Input: part model. Units: mm. Frame: model coordinates. A direction names the side the tool comes from. Give positions to 0.01 mm unless a question says otherwise; leave off trailing zeros. Write each loop counter-clockwise with the first axis right and the second up, starting at its lowest first coordinate (ties: lowest second). Pieces come first, ordered by that corner, then holes. Notation, with made-up numbers: (60, -21.75) - (118, -21.75) arc R23 ccw to (118, 8.25) - close; hole circle Ø3 at (54, -16.5). An arc over 180 degrees is marked (long way). Use a Markdown table: item, result. Add a question column.
1. Mould query, pull axis X, two halves, no side actions, for faces 6 (the flat face through (123, 28, 39)), 7 (the flat face through (103.5, 15, 0)), 8 (the cylindrical face through (25, 15, -31)). Classes: released by +X, released by -X, zero draft, split by the parting line, or undercut.
2. Section query D-D, the plane x = 56.5. Return loops of the section in (y, z).
3. Material intervals for probe 1 along Z at (x, y) = (79.5, 19.25); probe 2 along Z at (x, y) = (112, 23.5); probe 3 along Y at (x, z) = (31, -23), sorted ascending.
4. Section query A-A, the plane x = 110. Return loops of the section in (y, z).
5. Section query B-B, the plane y = 22.75. Return loops of the section in (x, z), plus the area to 3 significant figures.
6. Pin query (flat end, axial travel): pin 1 (4 mm diameter, centred on y = 23, z = 14.5, fed in from +X); pin 2 (9 mm diameter, centred on y = 25, z = 15, fed in from -X); pin 3 (10.5 mm diameter, centred on x = 56.5, z = -32, fed in from +Y); pin 4 (8 mm diameter, centred on x = 70, z = -30, fed in from +Y). Return the tip coordinate at first contact, or that it passes through.
7. Set-up query: faces 1 (the flat face through (71, 15, -48)), 2 (the flat face through (56, 15, 36.5)), 3 (the flat face through (105, 4, -39)), 4 (the flat face through (119, 26, -31)), 5 (the flat face through (119, 4, -31)). Return all of +Z, -Z, +X, -X, +Y, -Y with unobstructed straight access to the full face (end or side cutting, diameter ignored); none if empty.
8. Section query C-C, the plane z = -5.5. Return loops of the section in (x, y), plus the area to 3 significant figures.
```python
from build123d import *

# Parameters (mm, degrees)
BOSS_EXTRUDE1_DEPTH = 30
CUT_EXTRUDE1_DEPTH  = 2
CUT_EXTRUDE2_DEPTH  = 2
SKETCH5_W           = 6.5
SKETCH5_H           = 96
CUT_EXTRUDE3_DEPTH  = 11.5
CUT_EXTRUDE4_DEPTH  = 5.5
CUT_EXTRUDE5_DEPTH  = 5.5
SKETCH8_W           = 25
SKETCH8_H           = 30
CUT_EXTRUDE6_DEPTH  = 1
SKETCH9_W           = 25
SKETCH9_H           = 30
CUT_EXTRUDE7_DEPTH  = 0.5


with BuildPart() as part:
    # Sketch2 → Boss-Extrude1 (new body)
    # profile 1 of 3: a face of its own
    with BuildSketch(Plane(origin=(0, 0, 0), x_dir=(1, 0, 0), z_dir=(0, 1, 0))):
        Polygon((114.5, 12.5), (133, 31), (98, 31), (98, 48), (0, 48), (0, -48), (98, -48), (98, -31), (133, -31), (114.5, -12.5), (105, -12.5), (105, 12.5), align=None)
        with BuildLine():
            Line((81.5, -36.5), (30.5, -36.5))
            ThreePointArc((30.5, -36.5), (25, -31), (30.5, -25.5))
            Line((30.5, -25.5), (81.5, -25.5))
            ThreePointArc((81.5, -25.5), (87, -31), (81.5, -36.5))
        make_face(mode=Mode.SUBTRACT)
        with BuildLine():
            ThreePointArc((30.5, 25.5), (25, 31), (30.5, 36.5))
            Line((30.5, 36.5), (81.5, 36.5))
            ThreePointArc((81.5, 36.5), (87, 31), (81.5, 25.5))
            Line((81.5, 25.5), (30.5, 25.5))
        make_face(mode=Mode.SUBTRACT)
    # profile 2 of 3: a face of its own
    with BuildSketch(Plane(origin=(0, 0, 0), x_dir=(1, 0, 0), z_dir=(0, 1, 0))):
        Polygon((133, 31), (140, 38), (140, 48), (98, 48), (98, 31), align=None)
    # profile 3 of 3: a face of its own
    with BuildSketch(Plane(origin=(0, 0, 0), x_dir=(1, 0, 0), z_dir=(0, 1, 0))):
        Polygon((98, -31), (98, -48), (140, -48), (140, -38), (133, -31), align=None)
    extrude(amount=BOSS_EXTRUDE1_DEPTH)

    # Sketch3 → Cut-Extrude1 (cut)
    with BuildSketch(Plane(origin=(0, 30, 0), x_dir=(1, 0, 0), z_dir=(0, 1, 0))):
        Polygon((105, 48), (105, 31), (133, 31), (140, 38), (140, 48), align=None)
        Polygon((140, -38), (140, -48), (105, -48), (105, -31), (133, -31), align=None)
    extrude(amount=-CUT_EXTRUDE1_DEPTH, mode=Mode.SUBTRACT)

    # Sketch4 → Cut-Extrude2 (cut)
    with BuildSketch(Plane.XZ):
        Polygon((105, 48), (105, 31), (133, 31), (140, 38), (140, 48), align=None)
        Polygon((105, -48), (105, -31), (133, -31), (140, -38), (140, -48), align=None)
    extrude(amount=-CUT_EXTRUDE2_DEPTH, mode=Mode.SUBTRACT)

    # Sketch5 → Cut-Extrude3 (cut)
    with BuildSketch(Plane(origin=(0, 30, 0), x_dir=(1, 0, 0), z_dir=(0, 1, 0))):
        with Locations((3.25, 0)):
            Rectangle(SKETCH5_W, SKETCH5_H)
    extrude(amount=-CUT_EXTRUDE3_DEPTH, mode=Mode.SUBTRACT)

    # Sketch6 → Cut-Extrude4 (cut)
    with BuildSketch(Plane(origin=(0, 30, 0), x_dir=(1, 0, 0), z_dir=(0, 1, 0))):
        Polygon((105, 12.5), (6.5, 12.5), (6.5, 48), (105, 48), (105, 31), (133, 31), (114.5, 12.5), align=None)
        Polygon((105, -12.5), (6.5, -12.5), (6.5, -48), (105, -48), (105, -31), (133, -31), (114.5, -12.5), align=None)
    extrude(amount=-CUT_EXTRUDE4_DEPTH, mode=Mode.SUBTRACT)

    # Sketch7 → Cut-Extrude5 (cut)
    with BuildSketch(Plane.XZ):
        Polygon((105, 12.5), (6.5, 12.5), (6.5, -12.5), (105, -12.5), (114.5, -12.5), (133, -31), (105, -31), (105, -48), (0, -48), (0, 48), (105, 48), (105, 31), (133, 31), (114.5, 12.5), align=None)
    extrude(amount=-CUT_EXTRUDE5_DEPTH, mode=Mode.SUBTRACT)

    # Sketch8 → Cut-Extrude6 (cut)
    with BuildSketch(Plane(origin=(105, 0, 0), x_dir=(0, 0, -1), z_dir=(1, 0, 0))):
        with Locations((0, 15)):
            Rectangle(SKETCH8_W, SKETCH8_H)
    extrude(amount=-CUT_EXTRUDE6_DEPTH, mode=Mode.SUBTRACT)

    # Sketch9 → Cut-Extrude7 (cut)
    with BuildSketch(Plane(origin=(104, 0, 0), x_dir=(0, 0, -1), z_dir=(1, 0, 0))):
        with Locations((0, 15)):
            Rectangle(SKETCH9_W, SKETCH9_H)
    extrude(amount=-CUT_EXTRUDE7_DEPTH, mode=Mode.SUBTRACT)


solid = part.part
```
Result sheet:
| question | item | result |
|---|---|---|
| 1 | face 6 | zero draft |
| 1 | face 7 | released by +X |
| 1 | face 8 | undercut |
| 2 | outline | (0, -12.5) - (5.5, -12.5) - (5.5, -25.5) - (24.5, -25.5) - (24.5, -12.5) - (30, -12.5) - (30, 12.5) - (24.5, 12.5) - (24.5, 25.5) - (5.5, 25.5) - (5.5, 12.5) - (0, 12.5) - close; (5.5, -48) - (24.5, -48) - (24.5, -36.5) - (5.5, -36.5) - close; (5.5, 36.5) - (24.5, 36.5) - (24.5, 48) - (5.5, 48) - close |
| 3 | probe 1 | z = -48 to -36.5, -25.5 to 25.5, 36.5 to 48 |
| 3 | probe 2 | z = -48 to -12.5, 12.5 to 48 |
| 3 | probe 3 | y = 5.5 to 24.5 |
| 4 | outline | (2, -48) - (28, -48) - (28, -31) - (24.5, -31) - (24.5, -12.5) - (5.5, -12.5) - (5.5, -31) - (2, -31) - close; (2, 31) - (5.5, 31) - (5.5, 12.5) - (24.5, 12.5) - (24.5, 31) - (28, 31) - (28, 48) - (2, 48) - close |
| 5 | outline | (6.5, -48) - (140, -48) - (140, -38) - (114.5, -12.5) - (103.5, -12.5) - (103.5, 12.5) - (114.5, 12.5) - (140, 38) - (140, 48) - (6.5, 48) - close; hole (30.5, -36.5) - (81.5, -36.5) arc R5.5 ccw to (81.5, -25.5) - (30.5, -25.5) arc R5.5 ccw to start; hole (30.5, 25.5) - (81.5, 25.5) arc R5.5 ccw to (81.5, 36.5) - (30.5, 36.5) arc R5.5 ccw to start |
| 5 | area | 9,940 mm² |
| 6 | pin 1 | stops at x = 118.5 |
| 6 | pin 2 | stops at x = 6.5 |
| 6 | pin 3 | stops at y = 24.5 |
| 6 | pin 4 | passes through |
| 7 | face 1 | -Z, +X, -X, +Y, -Y |
| 7 | face 2 | +Y, -Y |
| 7 | face 3 | +Z, -Z, -X, -Y |
| 7 | face 4 | +X, -X, +Y |
| 7 | face 5 | +X, -X, -Y |
| 8 | outline | (0, 5.5) - (6.5, 5.5) - (6.5, 0) - (103.5, 0) - (103.5, 30) - (6.5, 30) - (6.5, 18.5) - (0, 18.5) - close |
| 8 | area | 2,990 mm² |
